Autodesk Inventor part; units mm, degrees
ref_plane "YZ Plane" through (0, 0, 0) normal (1, 0, 0) x (0, 1, 0)
ref_plane "XZ Plane" through (0, 0, 0) normal (0, 1, 0) x (-1, 0, 0)
ref_plane "XY Plane" through (0, 0, 0) normal (0, 0, 1) x (1, 0, 0)
sketch "Sketch1" plane through (0, 0, 0) normal (0, 0, 1) x (1, 0, 0)
  line L0 (0, 0) -> (2033.3333, 0)
  line L1 (2033.3333, 0) -> (2033.3333, 790)
  line L2 (2033.3333, 790) -> (0, 790)
  line L3 (0, 790) -> (0, 0)
  dimension "ancho" = 2033.3333
  dimension "d1" = 790
extrude "Extrusion1" add sketch "Sketch1" along normal blind 50
fillet "Fillet1" radius 50 1 edges at (1016.6667, 0, 50)
sketch "Sketch2" plane through (2033.3333, 790, 50) normal (1, 0, 0) x (0, 0, -1)
  line L0 (50, 0) -> (-50, 0)
  line L1 (-50, 0) -> (-50, 0)
  line L2 (-30, -20) -> (50, -20)
  line L3 (50, -20) -> (50, 0)
  arc A0 (-50, 0) -> (-30, -20) centre (-30, 0) ccw
  point P0 (50, -790)
  point P1 (-50, -20)
  dimension "d5" = 100
  dimension "d6" = 20
  dimension "d7" = 20
extrude "Extrusion2" add sketch "Sketch2" against normal up to surface (2033.3333 mm away)
properties part number "meson"
Design review of the part built by this model. Coordinates are the model's own, in mm. A direction names the side the tool comes from. Give positions to 0.01 mm unless a question says otherwise; leave off trailing zeros. Order: outer loops, then holes, each group sorted by start corner. A loop starts at its lowest first (then second) coordinate and runs counter-clockwise, first axis right, second up. Notation, with made-up numbers: (11.5, -17) -> (18.5, -17) arc R24 ccw to (18.5, 4) -> close; hole circle Ø11 at (73, -38). An arc over 180 degrees is marked (long way). Write each question's results on one line, items separated by ' | '. Start each with the question number.
Q1. Add section B-B on y = 239. Give the boundary of the cut face in (x, z), and give its area (3 significant figures).
Q2. For pin 1 (12 mm diameter, centred on x = 1297.5, y = 118, fed in from +Z); pin 2 (9 mm diameter, centred on x = 686.5, z = 65, fed in from -Y); pin 3 (1.5 mm diameter, centred on y = 650.5, z = 51, fed in from -X); pin 4 (12 mm diameter, centred on x = 332.5, z = 22.5, fed in from -Y), all flat-tipped, find the tip position at first contact; note any pin that passes through.
Q3. Wall thickness on L1, parallel to Z at x = 161, y = 469; L2, parallel to Y at x = 1214.5, z = 65; L3, parallel to Y at x = 1603, z = 21.5: over which ranges is each line inside the solid? List them lowest first. Write a range as from..to.
Q4. Machinability: for faces 1 (the flat face through (2033.333, 389, 27)), 2 (the flat face through (1002, 415, 50)), which of the approach directions +Z, -Z, +X, -X, +Y, -Y give a long, thin tool a straight path to every point of the face, cutting with its end or side? Answer none if there is none.
Found:
1) outline: (0, 0) -> (2033.33, 0) -> (2033.33, 50) -> (0, 50) -> close | area: 102,000 mm2
2) pin 1: stops at z = 50 | pin 2: stops at y = 770 | pin 3: passes through | pin 4: stops at y = 2.8
3) L1: z = 0..50 | L2: y = 770..790 | L3: y = 4.86..790
4) face 1: +Z, -Z, +X, +Y, -Y | face 2: +Z, +X, -X, -Y
